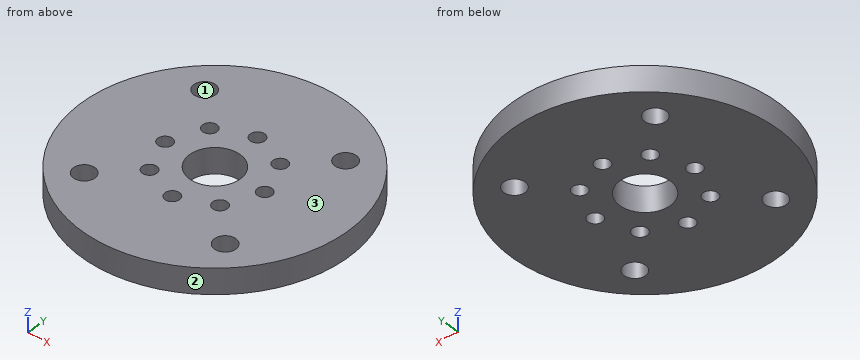
Solid Edge part; units mm, degrees
sketch "Sketch1" plane through (0, 0, 0) normal (0, 0, 1) x (1, 0, 0)
  circle A0 centre (0, 0) radius 21
  circle A1 centre (0, 0) radius 4
  circle A2 centre (8, 0) radius 1.15
  circle A3 centre (5.6569, 5.6569) radius 1.15
  circle A4 centre (0, 8) radius 1.15
  circle A5 centre (-5.6569, 5.6569) radius 1.15
  circle A6 centre (-8, 0) radius 1.15
  circle A7 centre (-5.6569, -5.6569) radius 1.15
  circle A8 centre (0, -8) radius 1.15
  circle A9 centre (5.6569, -5.6569) radius 1.15
  circle A10 centre (11.3137, 11.3137) radius 1.7
  circle A11 centre (-11.3137, 11.3137) radius 1.7
  circle A12 centre (-11.3137, -11.3137) radius 1.7
  circle A13 centre (11.3137, -11.3137) radius 1.7
extrude "Protrusion1" add sketch "Sketch1" along normal blind 4
Geometry: final body of the model. Coordinates: model frame, mm. Face numbers are marked on the shaded views. Coordinates: 2 decimals unless noted, no trailing zeros. Order: outer loops, then holes, each group sorted by start corner. A loop starts at its lowest first (then second) coordinate and runs counter-clockwise, first axis right, second up. Notation, with made-up numbers: (33.25, -34) -> (49.25, -34) arc R10 cw to (49.25, -21) -> close; hole circle Ø3 at (9, 20). An arc over 180 degrees is marked (long way). Answer in a Markdown table with one row per item.
Item 1: Contact query for flat-ended pins moving along their axis: P1, Ø2.5, axis at x = 0, y = -8, coming from the -Z side; P2, Ø2, axis at x = 14, z = 0.5, coming from the +Y side; P3, Ø1.5, axis at y = 13.5, z = 0.5, coming from the -X side. Output: stop coordinate, or through.
Return value:
| item | result |
|---|---|
| P1 | stops at z = 0 |
| P2 | stops at y = 16.49 |
| P3 | stops at x = -16.69 |
Item 2: Draft query along X for the marked faces 1, 2 and 3. Return one class per face: released by +X, released by -X, zero draft, split by the parting line, or undercut.
Return value:
| item | result |
|---|---|
| face 1 | undercut |
| face 2 | split by the parting line |
| face 3 | zero draft |
Item 3: Section D-D on x = 8. Output: boundary loops of the cut face in (y, z).
Return value:
| item | result |
|---|---|
| outline | (-19.42, 0) -> (-1.15, 0) -> (-1.15, 4) -> (-19.42, 4) -> close; (1.15, 0) -> (19.42, 0) -> (19.42, 4) -> (1.15, 4) -> close |
Item 4: Section A-A on x = 0. Output: boundary loops of the cut face in (y, z).
Return value:
| item | result |
|---|---|
| outline | (-21, 0) -> (-9.15, 0) -> (-9.15, 4) -> (-21, 4) -> close; (-6.85, 0) -> (-4, 0) -> (-4, 4) -> (-6.85, 4) -> close; (4, 0) -> (6.85, 0) -> (6.85, 4) -> (4, 4) -> close; (9.15, 0) -> (21, 0) -> (21, 4) -> (9.15, 4) -> close |
Item 5: Ray query, L1, parallel to Y at x = 0, z = 1.3; L2, parallel to Y at x = -6, z = 0.9; L3, parallel to X at y = -1, z = 2. Return the intervals inside material, ascending.
Return value:
| item | result |
|---|---|
| L1 | y = -21 to -9.15, -6.85 to -4, 4 to 6.85, 9.15 to 21 |
| L2 | y = -20.12 to -6.75, -4.56 to 4.56, 6.75 to 20.12 |
| L3 | x = -20.98 to -8.57, -7.43 to -3.87, 3.87 to 7.43, 8.57 to 20.98 |
Item 6: Section C-C on z = 1.3. State how many separate pieces and enclosed holes the cut face has, plus the area to 3 significant figures.
Return value:
| item | result |
|---|---|
| separate pieces | 1 |
| enclosed holes | 13 |
| area | 1,270 mm² |
